```python
from build123d import *

# Parameters (mm, degrees)
BASPROSKE_W        = 5
BASPROSKE_H        = 12
TOOTHCUT_DEPTH     = 18.691806013
TEETHCUTS_COUNT    = 10
TEETHCUTS_ANGLE    = 324
HUBNEAONESKE_R     = 6
HUBNEARONE_DEPTH   = 3.0000508
BORSKE_R           = 3
BORE_DEPTH         = 8.0000508
SKETCH1_R          = 3.5
SKETCH1_R_2        = 3
CUT_EXTRUDE1_DEPTH = 1


with BuildPart() as part:
    # BasProSke → Base-Revolve (revolve)
    with BuildSketch(Plane(origin=(0, 0, 0), x_dir=(1, 0, 0), z_dir=(0, 1, 0)), mode=Mode.PRIVATE) as base_revolve_sk:
        with Locations((2.5, 6)):
            Rectangle(BASPROSKE_W, BASPROSKE_H)
    revolve(base_revolve_sk.sketch.rotate(Axis((-10, 0, 0), (1, 0, 0)), 180), axis=Axis((-10, 0, 0), (1, 0, 0)))

    # TooCutSke → ToothCut (cut, through all)
    with BuildSketch(Plane(origin=(0, 0, 0), x_dir=(0, 0, -1), z_dir=(1, 0, 0))):
        with BuildLine():
            ThreePointArc((1.173662691, 7.406586048), (0, 7.499), (-1.173662691, 7.406586048))
            ThreePointArc((-1.173662691, 7.406586048), (-1.668191438, 9.834565786), (-3.497907776, 11.50542856))
            ThreePointArc((-3.497907776, 11.50542856), (0, 12.0254), (3.497907776, 11.50542856))
            ThreePointArc((3.497907776, 11.50542856), (1.668191438, 9.834565786), (1.173662691, 7.406586048))
        make_face()
    toothcut = extrude(amount=TOOTHCUT_DEPTH, mode=Mode.SUBTRACT)

    # TeethCuts: ToothCut ×10 about axis
    teethcuts_axis = Axis((-10, 0, 0), (1, 0, 0))
    for i in range(1, TEETHCUTS_COUNT):
        add(toothcut.rotate(teethcuts_axis, i * TEETHCUTS_ANGLE / (TEETHCUTS_COUNT - 1)), mode=Mode.SUBTRACT)

    # HubNeaOneSke → HubNearOne (add)
    with BuildSketch(Plane.ZY):
        with Locations(Location((0, 0, 0), (0, 0, 180))):
            Circle(HUBNEAONESKE_R)
    extrude(amount=HUBNEARONE_DEPTH)

    # BorSke → Bore (cut, symmetric)
    with BuildSketch(Plane(origin=(0, 0, 0), x_dir=(0, 0, -1), z_dir=(1, 0, 0))):
        with Locations(Location((0, 0, 0), (0, 0, 180))):
            Circle(BORSKE_R)
    extrude(amount=BORE_DEPTH, both=True, mode=Mode.SUBTRACT)

    # Sketch1 → Cut-Extrude1 (cut)
    with BuildSketch(Plane.ZY.offset(3.0000508)):
        Circle(SKETCH1_R)
        Circle(SKETCH1_R_2, mode=Mode.SUBTRACT)
    extrude(amount=-CUT_EXTRUDE1_DEPTH, mode=Mode.SUBTRACT)


solid = part.part
```
Can you work these out from the model? Positions are in its coordinate system, mm. Coordinates: 2 decimals unless noted, no trailing zeros. Loops run counter-clockwise (first coordinate to the right, second up) from the corner with the lowest first, then second, coordinate; pieces in that order, holes last. Notation, with made-up numbers: M 71.25,-16.75 L 115.25,-16.75 A13 ccw 115.25,-2.75 Z; hole C -21.75,13 d3. An arc over 180 degrees is marked long. Put each result on its own line as item: value. Start each with the question number.
(1) I need wall thicknesses on probe 1 along Y at (x, z) = (0.75, 0); probe 2 along X at (y, z) = (3.75, -5.5); probe 3 along Y at (x, z) = (-2.4, 0). Which ranges of each line are inside material? Lowest first, please.
(2) Imagine slicing it at A-A on z = 0. List the corners of the cut face in (x, y) for me, and give its area (3 significant figures).
(3) We'd pull the mould along Y, two halves only. Please class faces 1 (the face through (1.55, -0.9, 2.86)), 2 (the face through (-3, 3, -3)): +Y half, -Y half, draft (parallel to the pull), parting line (faces both ways), or undercut.
(4) Imagine slicing it at D-D on x = -2.5. List the corners of the cut face in (y, z) for me.
(5) Imagine slicing it at C-C on y = 8. List the corners of the cut face in (x, z) for me.
(6) Will these pins go through, and if not, where does the flat tip stop? pin 1 Ø1.5 at (x, y) = (3.5, 7) entering from +Z; pin 2 Ø4 at (x, z) = (-0.5, -7) entering from +Y; pin 3 Ø1.5 at (x, y) = (-0.5, 3.5) entering from -Z.
(7) Imagine slicing it at B-B on z = 7.75. List the corners of the cut face in (x, y) for me, and give its area (3 significant figures).
Worked answers:
1. probe 1: y = -7.5 to -3, 3 to 7.5
1. probe 2: x = 0 to 5
1. probe 3: y = -6 to -3.5, 3.5 to 6
2. outline: M -3,-6 L 0,-6 L 0,-7.5 L 5,-7.5 L 5,-3 L -2,-3 L -2,-3.5 L -3,-3.5 Z; M -3,3.5 L -2,3.5 L -2,3 L 5,3 L 5,7.5 L 0,7.5 L 0,6 L -3,6 Z
2. area: 62.0 mm2
3. face 1: undercut
3. face 2: draft
4. outline: C 0,0 d12; hole C 0,0 d7
5. outline: M 0,-4.21 L 5,-4.21 L 5,-1.15 L 0,-1.15 Z; M 0,1.15 L 5,1.15 L 5,4.21 L 0,4.21 Z
6. pin 1: stops at z = 9.86
6. pin 2: stops at y = 7.33
6. pin 3: stops at z = -8.2
7. outline: M 0,-7.2 L 5,-7.2 L 5,-3.79 L 0,-3.79 Z; M 0,-1.31 L 5,-1.31 L 5,1.31 L 0,1.31 Z; M 0,3.79 L 5,3.79 L 5,7.2 L 0,7.2 Z
7. area: 47.2 mm2
